```python
from build123d import *

# Parameters (mm, degrees)
ESQUISSE1_R                  = 57.5
BOSS_EXTRU_1_DEPTH           = 2
ESQUISSE2_R                  = 12
ENL_V_MAT_EXTRU_1_DEPTH      = 3
ESQUISSE5_W                  = 10
ESQUISSE5_H                  = 3
BOSS_EXTRU_3_DEPTH           = 21
ESQUISSE8_R                  = 2.5
ESQUISSE8_R_2                = 1
BOSS_EXTRU_4_DEPTH           = 5
ESQUISSE11_R                 = 3.5
ENL_V_MAT_EXTRU_7_DEPTH      = 84.985117729
ENL_V_MAT_EXTRU_8_DEPTH      = 84.985117729
ENL_V_MAT_EXTRU_8_DEPTH_BACK = 84.985117729
ESQUISSE12_R                 = 1.5
ESQUISSE14_R                 = 1
ENL_V_MAT_EXTRU_10_DEPTH     = 84.985117729


with BuildPart() as part:
    # Esquisse1 → Boss.-Extru.1 (new body)
    with BuildSketch(Plane(origin=(0, 0, 0), x_dir=(1, 0, 0), z_dir=(0, 1, 0))):
        with Locations(Location((0, 0, 0), (0, 0, 270))):
            Circle(ESQUISSE1_R)
    extrude(amount=BOSS_EXTRU_1_DEPTH)

    # Esquisse2 → Enlèv. mat.-Extru.1 (cut)
    with BuildSketch(Plane(origin=(0, 2, 0), x_dir=(1, 0, 0), z_dir=(0, 1, 0))):
        with Locations(Location((0, 0, 0), (0, 0, 270))):
            Circle(ESQUISSE2_R)
    extrude(amount=-ENL_V_MAT_EXTRU_1_DEPTH, mode=Mode.SUBTRACT)

    # Esquisse5 → Boss.-Extru.3 (add)
    with BuildSketch(Plane(origin=(0, 2, 0), x_dir=(1, 0, 0), z_dir=(0, 1, 0))):
        with Locations((0, -42.5)):
            Rectangle(ESQUISSE5_W, ESQUISSE5_H)
        with Locations((0, 42.5)):
            Rectangle(ESQUISSE5_W, ESQUISSE5_H)
    extrude(amount=BOSS_EXTRU_3_DEPTH)

    # Esquisse8 → Boss.-Extru.4 (add)
    # profile 1 of 2: a face of its own
    with BuildSketch(Plane(origin=(0, 2, 0), x_dir=(1, 0, 0), z_dir=(0, 1, 0))):
        with Locations(Location((27, 0, 0), (0, 0, 270))):
            Circle(ESQUISSE8_R)
        with Locations(Location((27, 0, 0), (0, 0, 270))):
            Circle(ESQUISSE8_R_2, mode=Mode.SUBTRACT)
    # profile 2 of 2: a face of its own
    with BuildSketch(Plane(origin=(0, 2, 0), x_dir=(1, 0, 0), z_dir=(0, 1, 0))):
        with Locations(Location((47, 0, 0), (0, 0, 270))):
            Circle(ESQUISSE8_R)
        with Locations(Location((47, 0, 0), (0, 0, 270))):
            Circle(ESQUISSE8_R_2, mode=Mode.SUBTRACT)
    extrude(amount=BOSS_EXTRU_4_DEPTH)

    # Esquisse11 → Enlèv. mat.-Extru.7 (cut, through all)
    with BuildSketch(Plane(origin=(0, 2, 0), x_dir=(1, 0, 0), z_dir=(0, 1, 0))):
        with Locations(Location((0, 31, 0), (0, 0, 270))):
            Circle(ESQUISSE11_R)
    extrude(amount=-ENL_V_MAT_EXTRU_7_DEPTH, mode=Mode.SUBTRACT)

    # Esquisse12 → Enlèv. mat.-Extru.8 (cut, two sides: drawn at the far end of the back side and taken through both)
    with BuildSketch(Plane(origin=(0, 2, 0), x_dir=(1, 0, 0), z_dir=(0, 1, 0)).offset(-ENL_V_MAT_EXTRU_8_DEPTH_BACK)):
        with Locations(Location((-27, 24, 0), (0, 0, 270))):
            Circle(ESQUISSE12_R)
        with Locations(Location((-27, -24, 0), (0, 0, 270))):
            Circle(ESQUISSE12_R)
    extrude(amount=ENL_V_MAT_EXTRU_8_DEPTH + ENL_V_MAT_EXTRU_8_DEPTH_BACK, mode=Mode.SUBTRACT)

    # Esquisse14 → Enlèv. mat.-Extru.10 (cut, through all)
    with BuildSketch(Plane(origin=(0, 2, 0), x_dir=(1, 0, 0), z_dir=(0, 1, 0))):
        with Locations(Location((34.5, -4.75, 0), (0, 0, 270))):
            Circle(ESQUISSE14_R)
        with Locations(Location((34.5, 4.75, 0), (0, 0, 270))):
            Circle(ESQUISSE14_R)
        with BuildLine():
            Line((11.01986842, -4.75), (13.01986842, -4.75))
            ThreePointArc((13.01986842, -4.75), (17.76986842, 0), (13.01986842, 4.75))
            Line((13.01986842, 4.75), (11.01986842, 4.75))
            Line((11.01986842, 4.75), (11.01986842, -4.75))
        make_face()
    extrude(amount=-ENL_V_MAT_EXTRU_10_DEPTH, mode=Mode.SUBTRACT)


solid = part.part
```
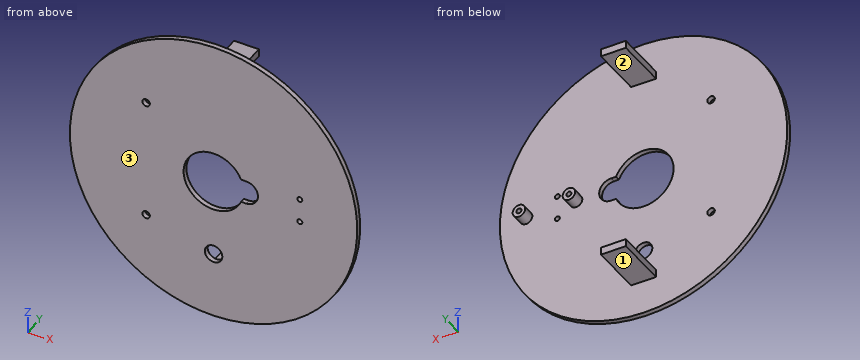
Read the model definition and answer for the solid it produces. Units are mm, in the model's axes. Face numbers are marked on the shaded views. A direction names the side the tool comes from. Coordinates: 2 decimals unless noted, no trailing zeros. Write each loop counter-clockwise with the first axis right and the second up, starting at its lowest first coordinate (ties: lowest second). Pieces come first, ordered by that corner, then holes. Notation, with made-up numbers: (85.5, 66.25) -> (96.5, 66.25) arc R15 ccw to (96.5, 71.25) -> close; hole circle Ø2 at (19, -31). An arc over 180 degrees is marked (long way). Return JSON: item names as keys, results as strings.
1. Each of these flat-tipped pins is pushed along its axis until it touches: P1, Ø1, axis at x = 12, y = 1, coming from the -Z side; P2, Ø12, axis at x = -20, y = 10, coming from the +Z side; P3, Ø3.5, axis at y = 8.5, z = -43, coming from the +X side; P4, Ø5.5, axis at x = 47, z = -0.5, coming from the +Y side. Where does it stop, or does it pass through?
Found:
{"P1": "z = -56.34", "P2": "through", "P3": "x = 5", "P4": "y = 7"}
2. A tool of negligible diameter and unlimited length cuts with its end or side. For the marked faces 1, 2 and 3, from which of +Z, -Z, +X, -X, +Y, -Y can it reach the whole face along a straight path? Write none if from no direction.
Found:
{"face 1": "-Z, +X, -X, +Y", "face 2": "+X, -X, +Y", "face 3": "+Z, -Z, +X, -X, -Y"}
3. Find the intervals of material crossed by line 1 along Z through (x, y) = (-27, 0.75); line 2 along X through (y, z) = (0.5, 0); line 3 along Z through (x, y) = (-2, 8), in increasing order. Write a range as from..to.
Found:
{"line 1": "-50.77..-25.5, -22.5..22.5, 25.5..50.77", "line 2": "-57.5..-12, 17.77..57.5", "line 3": "-44..-41, 41..44"}
4. A cutting plane is placed at C-C (z = -31). Determine the outline of the cut face in (x, y).
Found:
{"outline": "(-48.43, 0) -> (-3.5, 0) -> (-3.5, 2) -> (-48.43, 2) -> close; (3.5, 0) -> (48.43, 0) -> (48.43, 2) -> (3.5, 2) -> close"}
5. A cutting plane is placed at B-B (y = 8.5). Determine the outline of the cut face in (x, z).
Found:
{"outline": "(-5, -44) -> (5, -44) -> (5, -41) -> (-5, -41) -> close; (-5, 41) -> (5, 41) -> (5, 44) -> (-5, 44) -> close"}
6. A cutting plane is placed at A-A (x = 0). Determine the outline of the cut face in (y, z).
Found:
{"outline": "(0, -57.5) -> (2, -57.5) -> (2, -44) -> (23, -44) -> (23, -41) -> (2, -41) -> (2, -34.5) -> (0, -34.5) -> close; (0, -27.5) -> (2, -27.5) -> (2, -12) -> (0, -12) -> close; (0, 12) -> (2, 12) -> (2, 41) -> (23, 41) -> (23, 44) -> (2, 44) -> (2, 57.5) -> (0, 57.5) -> close"}
7. A cutting plane is placed at D-D (x = -27). Determine the outline of the cut face in (y, z).
Found:
{"outline": "(0, -50.77) -> (2, -50.77) -> (2, -25.5) -> (0, -25.5) -> close; (0, -22.5) -> (2, -22.5) -> (2, 22.5) -> (0, 22.5) -> close; (0, 25.5) -> (2, 25.5) -> (2, 50.77) -> (0, 50.77) -> close"}
